Verification items for the finished model (mm, model axes). Face numbers are marked on the shaded views. A direction names the side the tool comes from. Round coordinates to 2 decimals unless told otherwise and drop trailing zeros. Write each loop counter-clockwise with the first axis right and the second up, starting at its lowest first coordinate (ties: lowest second). Pieces come first, ordered by that corner, then holes. Notation, with made-up numbers: (50.5, 70) -> (92.5, 70) arc R33 cw to (92.5, 101) -> close; hole circle Ø6 at (45.5, -26.5). An arc over 180 degrees is marked (long way). Use CSV: the item, a comma, the result in double quotes.
Autodesk Inventor part; units mm, degrees
ref_plane "YZ Plane" through (0, 0, 0) normal (1, 0, 0) x (0, 1, 0)
ref_plane "XZ Plane" through (0, 0, 0) normal (0, 1, 0) x (-1, 0, 0)
ref_plane "XY Plane" through (0, 0, 0) normal (0, 0, 1) x (1, 0, 0)
sketch "Sketch1" plane through (0, 0, 0) normal (1, 0, 0) x (0, 1, 0)
  circle A0 centre (0, 0) radius 50
  dimension "d0" = 100
extrude "Extrusion1" add sketch "Sketch1" along normal blind 30
fillet "Fillet1" radius 5 2 edges at (30, -50, 0) (0, -50, 0)
sketch "Sketch2" plane through (30, 0, 0) normal (1, 0, 0) x (0, 0, -1)
  circle A0 centre (0, 0) radius 50
hole "Hole1" at (30, 0, 0) direction (-1, 0, 0) diameter 20 end through all
sketch "Sketch3" plane through (30, 0, 0) normal (1, 0, 0) x (0, 0, -1)
  circle A0 centre (0, 0) radius 25
  dimension "d11" = 50
extrude "Extrusion2" cut sketch "Sketch3" against normal blind 8.5
sketch "Sketch4" plane through (21.5, 0, 0) normal (1, 0, 0) x (0, 0, -1)
  line L0 (-7, -3) -> (-13, -3)
  line L1 (-13, -3) -> (-13, 3)
  line L2 (-13, 3) -> (-7, 3)
  line L3 (-7, 3) -> (-7, -3)
  circle A0 centre (0, 0) radius 10
  line L4 (-7, -3) -> (-13, 3) construction
  line L5 (-13, -3) -> (-7, 3) construction
  point P0 (-10, 0)
  dimension "d14" = 6
  dimension "d15" = 6
extrude "Extrusion3" cut sketch "Sketch4" against normal blind 28 contours L0 A0 L2 L3 | L0 L1 L2 A0 picked at (-7.9828, 0.338)
properties part number "100mm Traction Wheel StandIn" material "Rubber"
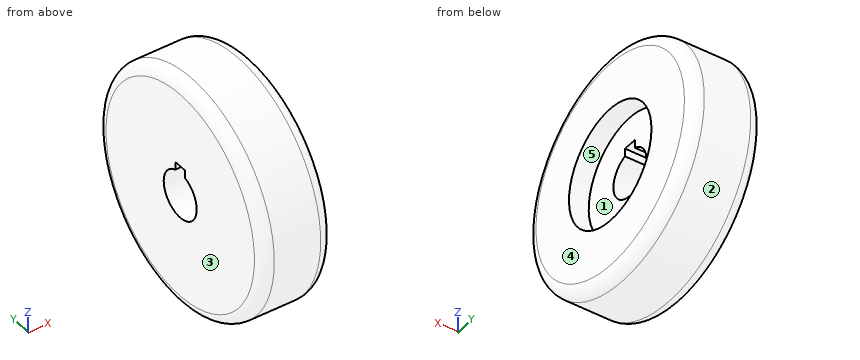
Q1. Mould release check, pull along Z, two halves, no side actions. Record for the marked faces 1, 2 and 3: released by +Z, released by -Z, zero draft, split by the parting line, or undercut.
Filled in:
face 1,"undercut"
face 2,"split by the parting line"
face 3,"zero draft"
Q2. Section check B-B (z = 0). Record the cut outline in (x, y).
Filled in:
outline,"(0, -45) arc R5 ccw to (5, -50) -> (25, -50) arc R5 ccw to (30, -45) -> (30, -25) -> (21.5, -25) -> (21.5, -10) -> (0, -10) -> close; (0, 10) -> (21.5, 10) -> (21.5, 25) -> (30, 25) -> (30, 45) arc R5 ccw to (25, 50) -> (5, 50) arc R5 ccw to (0, 45) -> close"
Q3. Section check A-A (y = 0). Record the cut outline in (x, z), plus the area to 3 significant figures.
Filled in:
outline,"(0, -45) arc R5 ccw to (5, -50) -> (25, -50) arc R5 ccw to (30, -45) -> (30, -25) -> (21.5, -25) -> (21.5, -10) -> (0, -10) -> close; (0, 13) -> (21.5, 13) -> (21.5, 25) -> (30, 25) -> (30, 45) arc R5 ccw to (25, 50) -> (5, 50) arc R5 ccw to (0, 45) -> close"
area,"2,060 mm²"
Q4. Section check C-C (x = 16). Record the cut outline in (y, z), plus the area to 3 significant figures.
Filled in:
outline,"circle Ø100 at (0, 0); hole (-3, 9.54) arc R10 ccw (long way) to (3, 9.54) -> (3, 13) -> (-3, 13) -> close"
area,"7,520 mm²"
Q5. Access from +Z, -Z, +X, -X, +Y, -Y to the whole of each face (thin tool, end or side, straight path). Record for the marked faces 4 and 5.
Filled in:
face 4,"+Z, -Z, +X, +Y, -Y"
face 5,"+X"
Q6. Go/stop test with flat-tipped pins: P1, Ø3, axis at x = 4.5, z = 34, coming from the -Y side; P2, Ø25, axis at y = 5.5, z = -10.5, coming from the +X side; P3, Ø4, axis at x = 9.5, z = 10.5, coming from the +Y side. Record where each tip stops, or that it passes through.
Filled in:
P1,"y = -37.97"
P2,"x = 21.5"
P3,"y = 49.27"
Q7. Material ranges on L1, parallel to Y at x = 9, z = 0.5; L2, parallel to Z at x = 11.5, y = 0; L3, parallel to Z at x = 24, y = -2, recorded low to high.
Filled in:
L1,"-50 to -9.99, 9.99 to 50"
L2,"-50 to -10, 13 to 50"
L3,"-49.96 to -24.92, 24.92 to 49.96"
